```python
from build123d import *

# Parameters (mm, degrees)
SKETCH1_W           = 7.366
SKETCH1_H           = 29.0322
BOSS_EXTRUDE1_DEPTH = 15.748
SKETCH2_W           = 2.54
SKETCH2_H           = 20.1422
CUT_EXTRUDE1_DEPTH  = 3.175
BOSS_EXTRUDE3_DEPTH = 1.5875


with BuildPart() as part:
    # Sketch1 → Boss-Extrude1 (new body)
    with BuildSketch(Plane(origin=(0, 0, 0), x_dir=(1, 0, 0), z_dir=(0, 1, 0))):
        Rectangle(SKETCH1_W, SKETCH1_H)
    extrude(amount=BOSS_EXTRUDE1_DEPTH)

    # Sketch2 → Cut-Extrude1 (cut)
    with BuildSketch(Plane(origin=(0, 15.748, 0), x_dir=(1, 0, 0), z_dir=(0, 1, 0))):
        with Locations((0, -1.905)):
            Rectangle(SKETCH2_W, SKETCH2_H)
    extrude(amount=-CUT_EXTRUDE1_DEPTH, mode=Mode.SUBTRACT)

    # Sketch5 → Boss-Extrude3 (add)
    with BuildSketch(Plane.XY.offset(14.5161)):
        with BuildLine():
            Line((-0.682666257, 6.414003725), (0.682666257, 6.414003725))
            ThreePointArc((0.682666257, 6.414003725), (1.254669982, 5.842), (0.682666257, 5.269996275))
            Line((0.682666257, 5.269996275), (-0.682666257, 5.269996275))
            ThreePointArc((-0.682666257, 5.269996275), (-1.254669982, 5.842), (-0.682666257, 6.414003725))
        make_face()
    extrude(amount=BOSS_EXTRUDE3_DEPTH)


solid = part.part
```
Verification items for the finished model (mm, model axes). A direction names the side the tool comes from. Give positions to 0.01 mm unless a question says otherwise; leave off trailing zeros. Order: outer loops, then holes, each group sorted by start corner. A loop starts at its lowest first (then second) coordinate and runs counter-clockwise, first axis right, second up. Notation, with made-up numbers: M 27,-13 L 76,-13 A14 cw 76,10 Z; hole C -15,-31 d5. An arc over 180 degrees is marked long. Return JSON: item names as keys, results as strings. Group by question number.
1) Section check B-B on z = -5. Record the cut outline in (x, y).
2) Mould release check, pull along Z, two halves, no side actions. Record for faces 4 (the face through (0, 8, 14.516)), 5 (the face through (0, 14, -8.166)), 6 (the face through (3.683, 8, 0)): pulls with the +Z half, pulls with the -Z half, needs draft (parallel to the pull), parting line crosses it, or undercut.
3) Section check C-C on x = 0. Record the cut outline in (y, z), and give its area (3 significant figures).
4) Section check A-A on y = 13.5. Record the cut outline in (x, z), and give its area (3 significant figures).
5) Section check D-D on y = 10.75. Record the cut outline in (x, z), and give its area (3 significant figures).
6) Access from +Z, -Z, +X, -X, +Y, -Y to the whole of each face (thin tool, end or side, straight path). Record for faces 1 (the face through (0, 12.573, 2)), 2 (the face through (1.255, 5.855, 15.299)), 3 (the face through (0, 6.414, 15)).
7) Go/stop test with flat-tipped pins: pin 1 Ø2 at (x, z) = (0, 6.5) entering from +Y; pin 2 Ø2 at (x, y) = (0, 9) entering from +Z. Record where each tip stops, or that it passes through.
8) Scan lines: line 1 (Y direction, x = -1, z = 11); line 2 (Z direction, x = -1, y = 11.5). Record each from-to range of solid material in increasing order.
Answer block:
{
 "1": {"outline": "M -3.68,0 L 3.68,0 L 3.68,15.75 L 1.27,15.75 L 1.27,12.57 L -1.27,12.57 L -1.27,15.75 L -3.68,15.75 Z"},
 "2": {"face 4": "pulls with the +Z half", "face 5": "undercut", "face 6": "needs draft"},
 "3": {"outline": "M 0,-14.52 L 15.75,-14.52 L 15.75,-8.17 L 12.57,-8.17 L 12.57,11.98 L 15.75,11.98 L 15.75,14.52 L 6.41,14.52 L 6.41,16.1 L 5.27,16.1 L 5.27,14.52 L 0,14.52 Z", "area": "395 mm^2"},
 "4": {"outline": "M -3.68,-14.52 L 3.68,-14.52 L 3.68,14.52 L -3.68,14.52 Z; hole M -1.27,-8.17 L 1.27,-8.17 L 1.27,11.98 L -1.27,11.98 Z", "area": "163 mm^2"},
 "5": {"outline": "M -3.68,-14.52 L 3.68,-14.52 L 3.68,14.52 L -3.68,14.52 Z", "area": "214 mm^2"},
 "6": {"face 1": "+Y", "face 2": "+Z, +X", "face 3": "+Z, +X, -X, +Y"},
 "7": {"pin 1": "stops at y = 12.57", "pin 2": "stops at z = 14.52"},
 "8": {"line 1": "y = 0 to 12.57", "line 2": "z = -14.52 to 14.52"}
}
